Work out the finished part from the listing and answer in its coordinate system (mm). Round coordinates to 2 decimals unless told otherwise and drop trailing zeros. Order: outer loops, then holes, each group sorted by start corner. A loop starts at its lowest first (then second) coordinate and runs counter-clockwise, first axis right, second up. Notation, with made-up numbers: (-1, 13) -> (27, 13) arc R13 ccw to (27, 33) -> close; hole circle Ø10 at (-18, -23). An arc over 180 degrees is marked (long way). Use a Markdown table: item, result. Add a question column.
Item 1: A cutting plane is placed at B-B, the plane y = 1.6. Give the number of separate pieces and of enclosed holes in the cut face, plus the area to 3 significant figures.
Item 2: Find the intervals of material crossed by L1, parallel to Z at x = 35, y = 1.6; L2, parallel to X at y = 1.5, z = 5.5; L3, parallel to Z at x = 42, y = 0.25, in increasing order. Write a range as [from, to].
Item 3: A cutting plane is placed at A-A, the plane x = 0. Determine the outline of the cut face in (y, z), plus the area to 3 significant figures.
Item 4: A cutting plane is placed at D-D, the plane x = 30.5. Determine the outline of the cut face in (y, z).
Item 5: A cutting plane is placed at C-C, the plane z = 37.5. Determine the outline of the cut face in (x, y).
Item 6: A flat-ended cylindrical pin translates along its axis: P1, Ø2.5, axis at x = 23.74, z = 13.71, coming from the +Y side. Find the tip coordinate at first contact, or state that the pin passes through.
from build123d import *

# Parameters (mm, degrees)
SKETCH2_R           = 1.5
BOSS_EXTRUDE1_DEPTH = 2
SKETCH3_R           = 51
SKETCH3_R_2         = 50
CUT_EXTRUDE1_DEPTH  = 1


with BuildPart() as part:
    # Sketch2 → Boss-Extrude1 (new body)
    with BuildSketch(Plane(origin=(0, 0, 0), x_dir=(1, 0, 0), z_dir=(0, 1, 0))):
        with BuildLine():
            ThreePointArc((-46.644081999, 29.14326019), (-55, 0), (-46.644081999, -29.14326019))
            ThreePointArc((-46.644081999, -29.14326019), (-45.124834326, -34.456279799), (-46.659212641, -39.764949504))
            ThreePointArc((-46.659212641, -39.764949504), (-45.961940777, -45.961940777), (-39.764949504, -46.659212641))
            ThreePointArc((-39.764949504, -46.659212641), (-34.456279799, -45.124834326), (-29.14326019, -46.644081999))
            ThreePointArc((-29.14326019, -46.644081999), (0, -55), (29.14326019, -46.644081999))
            ThreePointArc((29.14326019, -46.644081999), (34.456279799, -45.124834326), (39.764949504, -46.659212641))
            ThreePointArc((39.764949504, -46.659212641), (45.961940777, -45.961940777), (46.659212641, -39.764949504))
            ThreePointArc((46.659212641, -39.764949504), (45.124834326, -34.456279799), (46.644081999, -29.14326019))
            ThreePointArc((46.644081999, -29.14326019), (55, 0), (46.644081999, 29.14326019))
            ThreePointArc((46.644081999, 29.14326019), (45.124834326, 34.456279799), (46.659212641, 39.764949504))
            ThreePointArc((46.659212641, 39.764949504), (45.961940777, 45.961940777), (39.764949504, 46.659212641))
            ThreePointArc((39.764949504, 46.659212641), (34.456279799, 45.124834326), (29.14326019, 46.644081999))
            ThreePointArc((29.14326019, 46.644081999), (0, 55), (-29.14326019, 46.644081999))
            ThreePointArc((-29.14326019, 46.644081999), (-34.456279799, 45.124834326), (-39.764949504, 46.659212641))
            ThreePointArc((-39.764949504, 46.659212641), (-45.961940777, 45.961940777), (-46.659212641, 39.764949504))
            ThreePointArc((-46.659212641, 39.764949504), (-45.124834326, 34.456279799), (-46.644081999, 29.14326019))
        make_face()
        with Locations((-42.426406871, 42.426406871)):
            Circle(SKETCH2_R, mode=Mode.SUBTRACT)
        with Locations((-23.741169162, -13.706970407)):
            Circle(SKETCH2_R, mode=Mode.SUBTRACT)
        with Locations((23.741169162, -13.706970407)):
            Circle(SKETCH2_R, mode=Mode.SUBTRACT)
        with Locations((0, 27.413940814)):
            Circle(SKETCH2_R, mode=Mode.SUBTRACT)
        with Locations((42.426406871, 42.426406871)):
            Circle(SKETCH2_R, mode=Mode.SUBTRACT)
        with Locations((42.426406871, -42.426406871)):
            Circle(SKETCH2_R, mode=Mode.SUBTRACT)
        with Locations((-42.426406871, -42.426406871)):
            Circle(SKETCH2_R, mode=Mode.SUBTRACT)
    extrude(amount=BOSS_EXTRUDE1_DEPTH)

    # Sketch3 → Cut-Extrude1 (cut)
    with BuildSketch(Plane(origin=(0, 2, 0), x_dir=(1, 0, 0), z_dir=(0, 1, 0))):
        Circle(SKETCH3_R)
        Circle(SKETCH3_R_2, mode=Mode.SUBTRACT)
    extrude(amount=-CUT_EXTRUDE1_DEPTH, mode=Mode.SUBTRACT)


solid = part.part
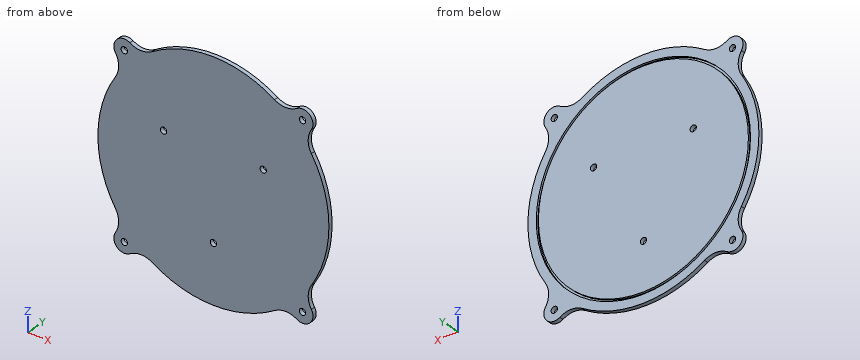
Reported:
| question | item | result |
|---|---|---|
| 1 | separate pieces | 2 |
| 1 | enclosed holes | 8 |
| 1 | area | 9,590 mm² |
| 2 | L1 | [-45.14, -37.09], [-35.71, 35.71], [37.09, 45.14] |
| 2 | L2 | [-54.72, -50.7], [-49.7, 49.7], [50.7, 54.72] |
| 2 | L3 | [-47.41, -43.86], [-40.99, 40.99], [43.86, 47.41] |
| 3 | outline | (0, -55) -> (2, -55) -> (2, -51) -> (1, -51) -> (1, -50) -> (2, -50) -> (2, -28.91) -> (0, -28.91) -> close; (0, -25.91) -> (2, -25.91) -> (2, 50) -> (1, 50) -> (1, 51) -> (2, 51) -> (2, 55) -> (0, 55) -> close |
| 3 | area | 212 mm² |
| 4 | outline | (0, -45.93) -> (2, -45.93) -> (2, -40.87) -> (1, -40.87) -> (1, -39.62) -> (2, -39.62) -> (2, 39.62) -> (1, 39.62) -> (1, 40.87) -> (2, 40.87) -> (2, 45.93) -> (0, 45.93) -> close |
| 5 | outline | (-45.6, 0) -> (45.6, 0) -> (45.6, 2) -> (34.57, 2) -> (34.57, 1) -> (33.07, 1) -> (33.07, 2) -> (-33.07, 2) -> (-33.07, 1) -> (-34.57, 1) -> (-34.57, 2) -> (-45.6, 2) -> close |
| 6 | P1 | through |
